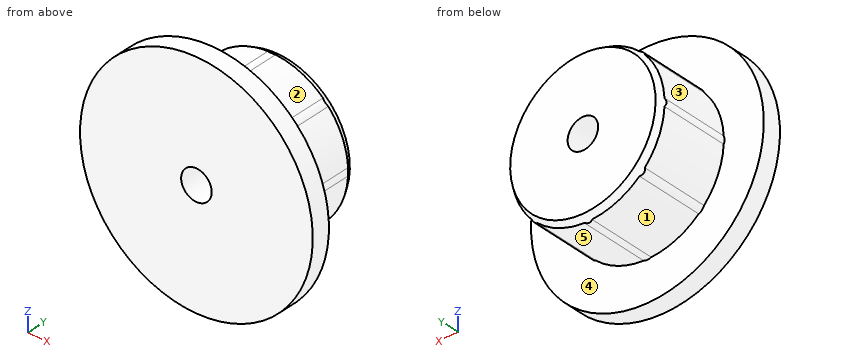
from build123d import *

# Parameters (mm, degrees)
BOSS_EXTRUDE1_DEPTH = 20
SKETCH3_R           = 30.48
BOSS_EXTRUDE2_DEPTH = 5
SKETCH11_R          = 4
CUT_EXTRUDE2_DEPTH  = 50.830320087


with BuildPart() as part:
    # Sketch1 → Boss-Extrude1 (new body)
    with BuildSketch(Plane(origin=(0, 0, 0), x_dir=(1, 0, 0), z_dir=(0, 1, 0))):
        with BuildLine():
            ThreePointArc((-1, 19.974984355), (-7.653668647, 18.47759065), (-13.417340111, 14.831553673))
            ThreePointArc((-13.417340111, 14.831553673), (-14.28355698, 14.28355698), (-14.831553673, 13.417340111))
            ThreePointArc((-14.831553673, 13.417340111), (-18.47759065, 7.653668647), (-19.974984355, 1))
            ThreePointArc((-19.974984355, 1), (-20.2, 0), (-19.974984355, -1))
            ThreePointArc((-19.974984355, -1), (-18.47759065, -7.653668647), (-14.831553673, -13.417340111))
            ThreePointArc((-14.831553673, -13.417340111), (-14.28355698, -14.28355698), (-13.417340111, -14.831553673))
            ThreePointArc((-13.417340111, -14.831553673), (-7.653668647, -18.47759065), (-1, -19.974984355))
            ThreePointArc((-1, -19.974984355), (0, -20.2), (1, -19.974984355))
            ThreePointArc((1, -19.974984355), (7.653668647, -18.47759065), (13.417340111, -14.831553673))
            ThreePointArc((13.417340111, -14.831553673), (14.28355698, -14.28355698), (14.831553673, -13.417340111))
            ThreePointArc((14.831553673, -13.417340111), (18.47759065, -7.653668647), (19.974984355, -1))
            ThreePointArc((19.974984355, -1), (20.2, 0), (19.974984355, 1))
            ThreePointArc((19.974984355, 1), (18.47759065, 7.653668647), (14.831553673, 13.417340111))
            ThreePointArc((14.831553673, 13.417340111), (14.28355698, 14.28355698), (13.417340111, 14.831553673))
            ThreePointArc((13.417340111, 14.831553673), (7.653668647, 18.47759065), (1, 19.974984355))
            ThreePointArc((1, 19.974984355), (0, 20.2), (-1, 19.974984355))
        make_face()
    extrude(amount=BOSS_EXTRUDE1_DEPTH)

    # Sketch2 → Cut-Revolve1 (revolve, cut)
    with BuildSketch(Plane.XY, mode=Mode.PRIVATE) as cut_revolve1_sk:
        Polygon((-18.61228676, 20.75), (-20.724984355, 17.090700423), (-20.724984355, 20.75), align=None)
    revolve(cut_revolve1_sk.sketch.rotate(Axis((0, 0, 0), (0, 1, 0)), 270), axis=Axis((0, 0, 0), (0, 1, 0)), mode=Mode.SUBTRACT)

    # Sketch3 → Boss-Extrude2 (add)
    with BuildSketch(Plane.XZ):
        with Locations(Location((0, 0, 0), (0, 0, 270))):
            Circle(SKETCH3_R)
    extrude(amount=BOSS_EXTRUDE2_DEPTH)

    # Sketch11 → Cut-Extrude2 (cut, through all)
    with BuildSketch(Plane(origin=(0, 20, 0), x_dir=(1, 0, 0), z_dir=(0, 1, 0))):
        with Locations(Location((0, 0, 0), (0, 0, 270))):
            Circle(SKETCH11_R)
    extrude(amount=-CUT_EXTRUDE2_DEPTH, mode=Mode.SUBTRACT)


solid = part.part
Read the model definition and answer for the solid it produces. Units are mm, in the model's axes. Face numbers are marked on the shaded views. A direction names the side the tool comes from. Coordinates: 2 decimals unless noted, no trailing zeros. Loops run counter-clockwise (first coordinate to the right, second up) from the corner with the lowest first, then second, coordinate; pieces in that order, holes last.
Q1. The part is cut by section D-D on z = -24. Write down the section's boundary in (x, y), and give its area (3 significant figures).
Q2. The part is cut by section B-B on z = 0. Write down the section's boundary in (x, y), and give its area (3 significant figures).
Q3. Each of these flat-tipped pins is pushed along its axis until it touches: pin 1 Ø4 at (y, z) = (4.5, -0.5) entering from +X; pin 2 Ø5 at (x, z) = (-0.5, 0.5) entering from +Y; pin 3 Ø2 at (x, y) = (-17.5, -0.5) entering from -Z; pin 4 Ø6 at (x, y) = (16, -1) entering from -Z. Where does it stop, or does it pass through?
Q4. Consider probe 1 along X at (y, z) = (14, 0); probe 2 along Y at (x, z) = (22, -1.5); probe 3 along X at (y, z) = (-1, -3.5). Determine where each line is inside the solid, lowest interval first.
Q5. Which of the six approach directions +Z, -Z, +X, -X, +Y, -Y give full straight-line access (tool end or side, diameter ignored) to the marked faces 1, 2, 3, 4 and 5?
Q6. The part is cut by section C-C on y = 4.75. Write down the section's boundary in (x, z).
Q7. The part is cut by section A-A on x = 0. Write down the section's boundary in (y, z), and give its area (3 significant figures).
Results below:
1. outline: (-18.79, -5) - (18.79, -5) - (18.79, 0) - (-18.79, 0) - close
1. area: 188 mm2
2. outline: (-30.48, -5) - (-4, -5) - (-4, 20) - (-19.05, 20) - (-20.2, 18) - (-20.2, 0) - (-30.48, 0) - close; (4, -5) - (30.48, -5) - (30.48, 0) - (20.2, 0) - (20.2, 18) - (19.05, 20) - (4, 20) - close
2. area: 910 mm2
3. pin 1: stops at x = 20.2
3. pin 2: passes through
3. pin 3: stops at z = -25.63
3. pin 4: stops at z = -27.57
4. probe 1: x = -20.2 to -4, 4 to 20.2
4. probe 2: y = -5 to 0
4. probe 3: x = -30.28 to -1.94, 1.94 to 30.28
5. face 1: -Z, -X, +Y
5. face 2: +Z, +X, +Y
5. face 3: +Z, -X, +Y
5. face 4: +Y
5. face 5: -Z, +X, +Y
6. outline: (-19.97, -1) arc R20 ccw to (-14.83, -13.42) arc R2.33 ccw to (-13.42, -14.83) arc R20 ccw to (-1, -19.97) arc R2.33 ccw to (1, -19.97) arc R20 ccw to (13.42, -14.83) arc R2.33 ccw to (14.83, -13.42) arc R20 ccw to (19.97, -1) arc R2.33 ccw to (19.97, 1) arc R20 ccw to (14.83, 13.42) arc R2.33 ccw to (13.42, 14.83) arc R20 ccw to (1, 19.97) arc R2.33 ccw to (-1, 19.97) arc R20 ccw to (-13.42, 14.83) arc R2.33 ccw to (-14.83, 13.42) arc R20 ccw to (-19.97, 1) arc R2.33 ccw to start; hole circle Ø8 at (0, 0)
7. outline: (-5, -30.48) - (0, -30.48) - (0, -20.2) - (18, -20.2) - (20, -19.05) - (20, -4) - (-5, -4) - close; (-5, 4) - (20, 4) - (20, 19.05) - (18, 20.2) - (0, 20.2) - (0, 30.48) - (-5, 30.48) - close
7. area: 910 mm2
